For this review, take the finished solid that the model builds, in its own axes (mm). Face numbers are marked on the shaded views. A direction names the side the tool comes from. Give positions to 0.01 mm unless a question says otherwise; leave off trailing zeros. Order: outer loops, then holes, each group sorted by start corner. A loop starts at its lowest first (then second) coordinate and runs counter-clockwise, first axis right, second up.
Item 1: Consider section B-B (z = 0). Give the boundary of the cut face in (x, y).
Item 2: For probe 1 along X at (y, z) = (-421.5, -0.5); probe 2 along X at (y, z) = (-492.5, 13); probe 3 along Z at (x, y) = (60.5, -711.2), list the stretches that pass through material, from the lowest coordinate up.
Item 3: The part is to be moulded in two halves that separate along Z. For the marked faces 1 and 2, say which applies: released by +Z, released by -Z, zero draft, split by the parting line, or undercut.
Item 4: Consider section D-D (x = 190.5). Give the boundary of the cut face in (y, z).
Item 5: Machinability: for the marked faces 3, 4 and 5, which of the approach directions +Z, -Z, +X, -X, +Y, -Y give a long, thin tool a straight path to every point of the face, cutting with its end or side? Answer none if there is none.
Item 6: For P1, Ø1, axis at x = 95, z = -20.5, coming from the -Y side; P2, Ø4, axis at x = 219, y = -534, coming from the -Z side; P3, Ø8, axis at x = 189, z = -13.5, coming from the +Y side, all flat-tipped, find the tip position at first contact; note any pin that passes through.
Item 7: Consider section A-A (y = -457.2). Give the boundary of the cut face in (x, z).
Item 8: Consider section C-C (y = -711.2). Give the boundary of the cut face in (x, z), plus the area to 3 significant figures.
```python
from build123d import *

# Parameters (mm, degrees)
SKETCH1_R   = 46.99
SKETCH1_R_2 = 44.45


with BuildPart() as part:
    # Sweep2: sweep along a curve in space
    with BuildLine() as sweep2_path:
        Line((0, 0, 0), (0, -711.2, 0))
        Line((0, -711.2, 0), (190.5, -711.2, 0))
        Line((190.5, -711.2, 0), (190.5, -457.2, 0))
        Line((190.5, -457.2, 0), (342.9, -457.2, 0))
    # Sketch1 → Sweep2 (sweep)
    with BuildSketch(Plane(origin=(0, 0, 0), x_dir=(1, 0, 0), z_dir=(0, 1, 0))):
        Circle(SKETCH1_R)
        Circle(SKETCH1_R_2, mode=Mode.SUBTRACT)
    sweep(path=sweep2_path.line, transition=Transition.RIGHT)


solid = part.part
```
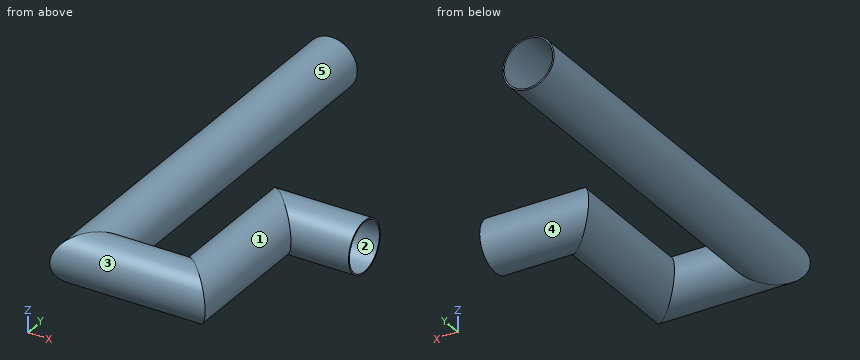
Resolved:
1. outline: (-46.99, -758.19) - (237.49, -758.19) - (237.49, -504.19) - (342.9, -504.19) - (342.9, -501.65) - (234.95, -501.65) - (234.95, -755.65) - (-44.45, -755.65) - (-44.45, 0) - (-46.99, 0) - close; (44.45, -666.75) - (146.05, -666.75) - (146.05, -412.75) - (342.9, -412.75) - (342.9, -410.21) - (143.51, -410.21) - (143.51, -664.21) - (46.99, -664.21) - (46.99, 0) - (44.45, 0) - close
2. probe 1: x = -46.99 to -44.45, 44.45 to 46.99, 143.51 to 146.05
2. probe 2: x = -45.16 to -42.51, 42.51 to 45.16, 145.34 to 147.99
2. probe 3: z = -46.99 to -44.45, 44.45 to 46.99
3. face 1: split by the parting line
3. face 2: undercut
4. outline: (-711.2, -46.99) - (-457.2, -46.99) arc R46.99 ccw to (-457.2, 46.99) - (-711.2, 46.99) arc R46.99 ccw to start; hole (-711.2, -44.45) - (-457.2, -44.45) arc R44.45 ccw to (-457.2, 44.45) - (-711.2, 44.45) arc R44.45 ccw to start
5. face 3: none
5. face 4: +X
5. face 5: +Y
6. P1: stops at y = -753.72
6. P2: stops at z = -38.8
6. P3: stops at y = -411.18
7. outline: circle Ø93.98 at (0, 0); (190.5, -46.99) - (342.9, -46.99) - (342.9, -44.45) - (190.5, -44.45) arc R44.45 cw to (190.5, 44.45) - (342.9, 44.45) - (342.9, 46.99) - (190.5, 46.99) arc R46.99 ccw to start; hole circle Ø88.9 at (0, 0)
8. outline: (0, -46.99) - (190.5, -46.99) arc R46.99 ccw to (190.5, 46.99) - (0, 46.99) arc R46.99 ccw to start; hole (0, -44.45) - (190.5, -44.45) arc R44.45 ccw to (190.5, 44.45) - (0, 44.45) arc R44.45 ccw to start
8. area: 1,700 mm2
